```python
from build123d import *

# Parameters (mm, degrees)
BOSS_EXTRUDE1_DEPTH = 262
CUT_EXTRUDE3_START  = -33
CUT_EXTRUDE3_DEPTH  = 33
SKETCH4_R           = 44.45
CUT_EXTRUDE4_DEPTH  = 78
SKETCH6_W           = 33
SKETCH6_H           = 59.34931139
CUT_EXTRUDE6_DEPTH  = 19
SKETCH7_R           = 5.5
CUT_EXTRUDE7_DEPTH  = 13


with BuildPart() as part:
    # Sketch1 → Boss-Extrude1 (new body)
    with BuildSketch(Plane.XY):
        with BuildLine():
            Line((0, 0), (-13, 0))
            Line((-13, 0), (-82, 32.051995773))
            Line((-82, 32.051995773), (-82, 82))
            ThreePointArc((-82, 82), (-57.982756057, 139.982756057), (0, 164))
            Line((0, 164), (0, 110.575))
            ThreePointArc((0, 110.575), (-28.575, 82), (0, 53.425))
            Line((0, 53.425), (0, 0))
        make_face()
    extrude(amount=BOSS_EXTRUDE1_DEPTH)

    # Sketch2 → Cut-Extrude3 (cut)
    with BuildSketch(Plane.XY.offset(262).offset(CUT_EXTRUDE3_START)):
        with BuildLine():
            Line((0, 53.425), (0, 0))
            Line((0, 0), (-13, 0))
            Line((-13, 0), (-82, 32.051995773))
            Line((-82, 32.051995773), (-82, 82))
            ThreePointArc((-82, 82), (-81.800252121, 87.720030847), (-81.201981637, 93.412194279))
            Line((-81.201981637, 93.412194279), (-65.430668922, 81.090294344))
            Line((-65.430668922, 81.090294344), (-14.946427946, 145.707176139))
            Line((-14.946427946, 145.707176139), (-30.71774066, 158.029076074))
            ThreePointArc((-30.71774066, 158.029076074), (-15.646337621, 162.493429043), (0, 164))
            Line((0, 164), (0, 110.575))
            ThreePointArc((0, 110.575), (-28.575, 82), (0, 53.425))
        make_face()
    extrude(amount=CUT_EXTRUDE3_DEPTH, mode=Mode.SUBTRACT)

    # Sketch4 → Cut-Extrude4 (cut)
    with BuildSketch(Plane.XY.offset(229)):
        with Locations((0, 82)):
            Circle(SKETCH4_R)
    extrude(amount=-CUT_EXTRUDE4_DEPTH, mode=Mode.SUBTRACT)

    # Sketch6 → Cut-Extrude6 (cut)
    with BuildSketch(Plane(origin=(0, 0, 0), x_dir=(0, 0, -1), z_dir=(1, 0, 0))):
        with Locations((-54.5, 134.325344305)):
            Rectangle(SKETCH6_W, SKETCH6_H)
    extrude(amount=-CUT_EXTRUDE6_DEPTH, mode=Mode.SUBTRACT)

    # Sketch7 → Cut-Extrude7 (cut)
    with BuildSketch(Plane(origin=(0, 0, 0), x_dir=(0, 0, -1), z_dir=(1, 0, 0))):
        with BuildLine():
            ThreePointArc((-108.5, 26), (-110.110912703, 22.110912703), (-114, 20.5))
            Line((-114, 20.5), (0, 20.5))
            Line((0, 20.5), (0, 31.5))
            Line((0, 31.5), (-114, 31.5))
            ThreePointArc((-114, 31.5), (-110.110912703, 29.889087297), (-108.5, 26))
        make_face()
        with Locations((-114, 26)):
            Circle(SKETCH7_R)
    extrude(amount=-CUT_EXTRUDE7_DEPTH, mode=Mode.SUBTRACT)


solid = part.part
```
Part model, mm, in its own coordinate system. A direction names the side the tool comes from. Round coordinates to 2 decimals unless told otherwise and drop trailing zeros. Write each loop counter-clockwise with the first axis right and the second up, starting at its lowest first coordinate (ties: lowest second). Pieces come first, ordered by that corner, then holes. Notation, with made-up numbers: M 30.25,34.25 L 37.25,34.25 A19 ccw 37.25,58.25 Z; hole C 73.5,-25.5 d11. An arc over 180 degrees is marked long. Answer as CSV lines item,"result". Start each with the question number.
1) Drill centre lines: L1, parallel to Z at x = -11, y = 48.5; L2, parallel to Z at x = -10.5, y = 136.5; L3, parallel to Z at x = -33, y = 13.5. Where is each one in solid material? Low to high.
2) Mould opens along Z. For faces 6 (the face through (-6, 20.5, 58)), 7 (the face through (-19, 134, 55)), 8 (the face through (-32, 83, 151)) say: +Z half, -Z half, draft (parallel to the pull), parting line (faces both ways), or undercut.
3) Band-saw the part on B-B (x = -9.5). List the corners of the cut face in (y, z), then the cut area to 3 significant figures.
4) Drop flat-ended pins along their axis: pin 1 (16.5 mm diameter, centred on y = 122.5, z = 49, fed in from +X); pin 2 (6 mm diameter, centred on x = -69.5, z = 101, fed in from +Y); pin 3 (3 mm diameter, centred on x = -44.5, z = 227, fed in from -Y). Give the stop position or say it passes through.
5) Which spindle directions (+Z, -Z, +X, -X, +Y, -Y) get a long thin tool onto all of the face, cutting with end or side? Do faces 1 (the face through (-6.4, 26.1, 119.5)), 2 (the face through (-9, 134, 71)), 3 (the face through (-44.44, 82.98, 190.55)), 4 (the face through (-23, 152, 245)), 5 (the face through (-58.62, 139.34, 129.17)). Say none if no direction does.
6) Band-saw the part on A-A (z = 47). List the corners of the cut face in (x, y) (3 decimals), then the cut area to 3 significant figures.
7) Band-saw the part on D-D (y = 138). List the corners of the cut face in (x, z), then the cut area to 3 significant figures.
8) Band-saw the part on C-C (x = -23). List the corners of the cut face in (y, z), then the cut area to 3 significant figures.
Worked out:
1,L1,"0 to 151"
1,L2,"0 to 38, 71 to 229"
1,L3,"0 to 229"
2,face 6,"draft"
2,face 7,"undercut"
2,face 8,"+Z half"
3,outline,"M 0,0 L 20.5,0 L 20.5,114 A5.5 cw 31.5,114 L 31.5,0 L 55.05,0 L 55.05,151 L 38.58,151 L 38.58,229 L 0,229 Z; M 108.95,0 L 163.45,0 L 163.45,38 L 108.95,38 Z; M 108.95,71 L 163.45,71 L 163.45,229 L 125.42,229 L 125.42,151 L 108.95,151 Z"
3,area,"19,400 mm²"
4,pin 1,"x = -19"
4,pin 2,"y = 129.98"
4,pin 3,"y = 13.94"
5,face 1,"-Z, +X"
5,face 2,"+X, +Y"
5,face 3,"+Z, +X"
5,face 4,"+Z, +X, +Y"
5,face 5,"+Z, -Z, -X, +Y"
6,outline,"M -82,32.052 L -13,0 L 0,0 L 0,20.5 L -13,20.5 L -13,31.5 L 0,31.5 L 0,53.425 A28.575 cw -17.421,104.651 L -19,104.651 L -19,161.768 A82 ccw -82,82 Z"
6,area,"8,430 mm²"
7,outline,"M -59.9,0 L 0,0 L 0,38 L -19,38 L -19,71 L 0,71 L 0,229 L -20.97,229 L -20.97,262 L -59.9,262 Z"
7,area,"14,400 mm²"
8,outline,"M 4.65,0 L 65.04,0 L 65.04,151 L 43.96,151 L 43.96,229 L 4.65,229 Z; M 98.96,0 L 160.71,0 L 160.71,229 L 152,229 L 152,262 L 135.4,262 L 135.4,229 L 120.04,229 L 120.04,151 L 98.96,151 Z"
8,area,"25,200 mm²"
